Verification items for the finished model (mm, model axes). A direction names the side the tool comes from. Round coordinates to 2 decimals unless told otherwise and drop trailing zeros. Write each loop counter-clockwise with the first axis right and the second up, starting at its lowest first coordinate (ties: lowest second). Pieces come first, ordered by that corner, then holes. Notation, with made-up numbers: M 16,44 L 62,44 A34 ccw 62,76 Z; hole C -27.5,42 d11. An arc over 180 degrees is marked long. Answer in a Markdown table with one row per item. Add a question column.
1. Sectioned sample at D-D on y = 1. Record the cut outline in (x, z).
2. Sectioned sample at A-A on y = 15.25. Record the cut outline in (x, z).
3. Draft check along Y on faces 5 (the flat face through (0, 19, -1)), 6 (the flat face through (-6.844, 21, -1)), 7 (the flat face through (0, 17.3, 1)). Enter one of: pulls with the +Y half, pulls with the -Y half, needs draft (parallel to the pull), parting line crosses it, or undercut.
4. Sectioned sample at B-B on x = -1. Record the cut outline in (y, z).
5. Set-up check for faces 1 (the flat face through (6.844, 21, -1)), 2 (the flat face through (0, 24, 0)), 3 (the flat face through (-0.1, 0, 0.2)), 4 (the flat face through (4.1, 15, 1)): record each of +Z, -Z, +X, -X, +Y, -Y from which the full face is reachable in a straight line by a thin tool's end or side.
6. Material ranges on probe 1 along Y at (x, z) = (1.5, 0.8); probe 2 along X at (y, z) = (15.5, 1.65); probe 3 along X at (y, z) = (23, -0.45), recorded low to high.
7. Go/stop test with flat-tipped pins: pin 1 Ø1 at (x, y) = (3.5, 18) entering from +Z; pin 2 Ø4 at (x, y) = (4, 7) entering from -Z; pin 3 Ø1 at (y, z) = (19.5, 0) entering from +X. Record where each tip stops, or that it passes through.
8. Sectioned sample at C-C on y = 19.75. Record the cut outline in (x, z).
```python
from build123d import *
from build123d.topology import SkipClean

# Parameters (mm, degrees)
EXTRUDE_1_DEPTH          = 24
CUT_EXTRUDE_2_DEPTH      = 5
CUT_EXTRUDE_2_DEPTH_BACK = 5
EXTRUDE_2_DEPTH          = 24
EXTRUDE_START            = 2
EXTRUDE_3_DEPTH          = 2
EXTRUDE_4_DEPTH          = 2
CUT_EXTRUDE_3_DEPTH      = 13.65
FILLET_1_R               = 1
CUT_EXTRUDE_START        = -8
CUT_EXTRUDE_5_DEPTH      = 14
EXTRUDE_START_2          = -5
EXTRUDE_5_DEPTH          = 5
CUT_EXTRUDE_START_2      = -1.49247673
CUT_EXTRUDE_6_DEPTH      = 1.49247673


with BuildPart() as part:
    # Эскиз1 → Бобышка-Вытянуть1 (new body)
    with BuildSketch(Plane(origin=(0, 0, 0), x_dir=(1, 0, 0), z_dir=(0, 1, 0))):
        with BuildLine():
            Line((-6.84384702, 0.49247673), (-7.158835795, -1.684856977))
            ThreePointArc((-7.158835795, -1.684856977), (0, -2.2), (7.158835795, -1.684856977))
            Line((7.158835795, -1.684856977), (6.84384702, 0.49247673))
            ThreePointArc((6.84384702, 0.49247673), (0, 0), (-6.84384702, 0.49247673))
        make_face()
    extrude(amount=EXTRUDE_1_DEPTH)

    # Эскиз2 → Вырез-Вытянуть2 (cut, two sides: drawn at the far end of the back side and taken through both)
    with BuildSketch(Plane.XY.offset(-CUT_EXTRUDE_2_DEPTH_BACK)):
        with BuildLine():
            Line((3.05, 17.3), (-3.05, 17.3))
            ThreePointArc((-3.05, 17.3), (-3.169210201, 17.269768771), (-3.259607324, 17.186381965))
            Line((-3.259607324, 17.186381965), (-4.059452109, 15.958486928))
            ThreePointArc((-4.059452109, 15.958486928), (-4.089648868, 15.893165149), (-4.1, 15.821949749))
            Line((-4.1, 15.821949749), (-4.1, 14.788048333))
            Line((-4.1, 14.788048333), (-4.1, 14.3))
            Line((-4.1, 14.3), (4.1, 14.3))
            Line((4.1, 14.3), (4.1, 14.788048333))
            Line((4.1, 14.788048333), (4.1, 15.821949749))
            ThreePointArc((4.1, 15.821949749), (4.089648868, 15.893165149), (4.059452109, 15.958486928))
            Line((4.059452109, 15.958486928), (3.259607324, 17.186381965))
            ThreePointArc((3.259607324, 17.186381965), (3.169210201, 17.269768771), (3.05, 17.3))
        make_face()
        with BuildLine():
            Line((-0.063165968, 22.35), (1.436834032, 22.35))
            ThreePointArc((1.436834032, 22.35), (2.436834032, 21.35), (1.436834032, 20.35))
            Line((1.436834032, 20.35), (-1.563165968, 20.35))
            ThreePointArc((-1.563165968, 20.35), (-2.563165968, 21.35), (-1.563165968, 22.35))
            Line((-1.563165968, 22.35), (-0.063165968, 22.35))
        make_face()
    extrude(amount=CUT_EXTRUDE_2_DEPTH + CUT_EXTRUDE_2_DEPTH_BACK, mode=Mode.SUBTRACT)

    # Эскиз3 → Бобышка-Вытянуть2 (add)
    with BuildSketch(Plane(origin=(0, 24, 0), x_dir=(1, 0, 0), z_dir=(0, 1, 0))):
        with BuildLine():
            Line((-8.001110971, -0.035470346), (-8.100093787, -0.627249361))
            ThreePointArc((-8.100093787, -0.627249361), (-7.565495415, -0.713640135), (-7.029976751, -0.794129552))
            Line((-7.029976751, -0.794129552), (-6.944070721, -0.200311268))
            ThreePointArc((-6.944070721, -0.200311268), (-7.473045369, -0.120805428), (-8.001110971, -0.035470346))
        make_face()
        with BuildLine():
            Line((8.001110971, -0.035470346), (8.100093787, -0.627249361))
            ThreePointArc((8.100093787, -0.627249361), (7.565495415, -0.713640135), (7.029976751, -0.794129552))
            Line((7.029976751, -0.794129552), (6.944070721, -0.200311268))
            ThreePointArc((6.944070721, -0.200311268), (7.473045369, -0.120805428), (8.001110971, -0.035470346))
        make_face()
    extrude(amount=-EXTRUDE_2_DEPTH)

    # Эскиз4 → Бобышка-Вытянуть3 (add)
    with SkipClean():  # the faces are left unmerged after this step: merging them gives an invalid solid
        with BuildSketch(Plane(origin=(0, 24, 0), x_dir=(1, 0, 0), z_dir=(0, 1, 0)).offset(EXTRUDE_START)):
            with BuildLine():
                Line((-8.001110971, -0.035470346), (-8.100093787, -0.627249361))
                ThreePointArc((-8.100093787, -0.627249361), (0, -1.3), (8.100093787, -0.627249361))
                Line((8.100093787, -0.627249361), (8.001110971, -0.035470346))
                ThreePointArc((8.001110971, -0.035470346), (0, -0.7), (-8.001110971, -0.035470346))
            make_face()
        extrude(amount=-EXTRUDE_3_DEPTH)

    # Эскиз5 → Бобышка-Вытянуть4 (add)
    with SkipClean():  # the faces are left unmerged after this step: merging them gives an invalid solid
        with BuildSketch(Plane.XZ):
            with BuildLine():
                Line((8.001110971, 0.035470346), (8.100093787, 0.627249361))
                ThreePointArc((8.100093787, 0.627249361), (0, 1.3), (-8.100093787, 0.627249361))
                Line((-8.100093787, 0.627249361), (-8.001110971, 0.035470346))
                ThreePointArc((-8.001110971, 0.035470346), (0, 0.7), (8.001110971, 0.035470346))
            make_face()
        extrude(amount=EXTRUDE_4_DEPTH)

    # Эскиз6 → Вырез-Вытянуть3 (cut)
    with SkipClean():  # the faces are left unmerged after this step: merging them gives an invalid solid
        with BuildSketch(Plane.XZ):
            with BuildLine():
                Line((-7.158835795, 1.684856977), (-7.130200452, 1.486917549))
                ThreePointArc((-7.130200452, 1.486917549), (0, 2), (7.130200452, 1.486917549))
                Line((7.130200452, 1.486917549), (7.158835795, 1.684856977))
                ThreePointArc((7.158835795, 1.684856977), (0, 2.2), (-7.158835795, 1.684856977))
            make_face()
        extrude(amount=-CUT_EXTRUDE_3_DEPTH, mode=Mode.SUBTRACT)

    # Скругление1
    fillet_1_edges = [part.edges().sort_by_distance(p)[0] for p in [
        (7.144518124, 13.65, 1.585887263),
        (-7.144518124, 13.65, 1.585887263),
    ]]
    fillet(fillet_1_edges, radius=FILLET_1_R)

    # Эскиз8 → Вырез-Вытянуть5 (cut)
    with SkipClean():  # the faces are left unmerged after this step: merging them gives an invalid solid
        with BuildSketch(Plane(origin=(0, 26, 0), x_dir=(1, 0, 0), z_dir=(0, 1, 0)).offset(CUT_EXTRUDE_START)):
            with BuildLine():
                Line((8.100093787, -0.627249361), (8.001110971, -0.035470346))
                ThreePointArc((8.001110971, -0.035470346), (7.473045369, -0.120805428), (6.944070721, -0.200311268))
                Line((6.944070721, -0.200311268), (7.029976751, -0.794129552))
                ThreePointArc((7.029976751, -0.794129552), (7.565495415, -0.713640135), (8.100093787, -0.627249361))
            make_face()
            with BuildLine():
                Line((-8.001110971, -0.035470346), (-8.100093787, -0.627249361))
                ThreePointArc((-8.100093787, -0.627249361), (-7.565495415, -0.713640135), (-7.029976751, -0.794129552))
                Line((-7.029976751, -0.794129552), (-6.944070721, -0.200311268))
                ThreePointArc((-6.944070721, -0.200311268), (-7.473045369, -0.120805428), (-8.001110971, -0.035470346))
            make_face()
        extrude(amount=-CUT_EXTRUDE_5_DEPTH, mode=Mode.SUBTRACT)

    # Эскиз9 → Бобышка-Вытянуть5 (add)
    with SkipClean():  # the faces are left unmerged after this step: merging them gives an invalid solid
        with BuildSketch(Plane(origin=(0, 24, 0), x_dir=(1, 0, 0), z_dir=(0, 1, 0)).offset(EXTRUDE_START_2)):
            with BuildLine():
                Line((-6.84384702, 0.49247673), (-6.84384702, 1.49247673))
                Line((-6.84384702, 1.49247673), (6.84384702, 1.49247673))
                Line((6.84384702, 1.49247673), (6.84384702, 0.49247673))
                ThreePointArc((6.84384702, 0.49247673), (0, 0), (-6.84384702, 0.49247673))
            make_face()
        extrude(amount=EXTRUDE_5_DEPTH)

    # Эскиз10 → Вырез-Вытянуть6 (cut)
    with SkipClean():  # the faces are left unmerged after this step: merging them gives an invalid solid
        with BuildSketch(Plane.XY.offset(CUT_EXTRUDE_START_2)):
            with BuildLine():
                Line((1.436834032, 20.35), (-1.563165968, 20.35))
                ThreePointArc((-1.563165968, 20.35), (-2.563165968, 21.35), (-1.563165968, 22.35))
                Line((-1.563165968, 22.35), (1.436834032, 22.35))
                ThreePointArc((1.436834032, 22.35), (2.436834032, 21.35), (1.436834032, 20.35))
            make_face()
        extrude(amount=CUT_EXTRUDE_6_DEPTH, mode=Mode.SUBTRACT)


solid = part.part
```
Geometry check:
| question | item | result |
|---|---|---|
| 1 | outline | M -8.1,0.63 L -8,0.04 A48.5 cw -6.94,0.2 L -6.84,-0.49 A47.8 cw 6.84,-0.49 L 6.94,0.2 A48.5 cw 8,0.04 L 8.1,0.63 A49.1 ccw 7.03,0.79 L 7.13,1.49 A49.8 ccw -7.13,1.49 L -7.03,0.79 A49.1 ccw Z |
| 2 | outline | M -7.16,1.68 L -6.84,-0.49 A47.8 cw -4.1,-0.18 L -4.1,2.03 A50 ccw Z; M 4.1,-0.18 A47.8 cw 6.84,-0.49 L 7.16,1.68 A50 ccw 4.1,2.03 Z |
| 3 | face 5 | pulls with the -Y half |
| 3 | face 6 | needs draft |
| 3 | face 7 | undercut |
| 4 | outline | M -2,0.69 L 0,0.69 L 0,-0.01 L 14.3,-0.01 L 14.3,2.19 L 13.65,2.19 L 13.65,1.99 L 0,1.99 L 0,1.29 L -2,1.29 Z; M 17.3,-0.01 L 19,-0.01 L 19,-1.49 L 20.35,-1.49 L 20.35,2.19 L 17.3,2.19 Z; M 22.35,-1.49 L 24,-1.49 L 24,0.69 L 26,0.69 L 26,1.29 L 24,1.29 L 24,2.19 L 22.35,2.19 Z |
| 5 | face 1 | -Z, +X, +Y, -Y |
| 5 | face 2 | -Z, +Y |
| 5 | face 3 | -Z, -Y |
| 5 | face 4 | +Z, -Z |
| 6 | probe 1 | y = -2 to 14.3, 17.3 to 20.35, 22.35 to 26 |
| 6 | probe 2 | x = -7.15 to -4.1, 4.1 to 7.15 |
| 6 | probe 3 | x = -6.85 to 6.85 |
| 7 | pin 1 | stops at z = 2.11 |
| 7 | pin 2 | stops at z = -0.38 |
| 7 | pin 3 | stops at x = 8.08 |
| 8 | outline | M -8.1,0.63 L -8,0.04 A48.5 cw -6.94,0.2 L -6.84,-0.49 L -6.84,-1.49 L 6.84,-1.49 L 6.84,-0.49 L 6.94,0.2 A48.5 cw 8,0.04 L 8.1,0.63 A49.1 ccw 7.03,0.79 L 7.16,1.68 A50 ccw -7.16,1.68 L -7.03,0.79 A49.1 ccw Z |
